from build123d import *

# Parameters (mm, degrees)
SKETCH2_R           = 6
SKETCH4_R           = 8
BOSS_EXTRUDE1_DEPTH = 2
SKETCH5_R           = 8
SKETCH5_R_2         = 6
BOSS_EXTRUDE2_DEPTH = 2


with BuildPart() as part:
    # Sweep1: sweep along a curve in space
    with BuildLine() as sweep1_path:
        Line((0, 0, 0), (0, 0, 20))
        ThreePointArc((-10, 0, 30), (-2.928932188, 0, 27.071067812), (0, 0, 20))
        Line((-10, 0, 30), (-96, 0, 30))
    # Sketch2 → Sweep1 (sweep)
    with BuildSketch(Plane.XY):
        Circle(SKETCH2_R)
    sweep(path=sweep1_path.line)

    # Sketch4 → Boss-Extrude1 (add)
    with BuildSketch(Plane(origin=(0, 0, 0), x_dir=(-1, 0, 0), z_dir=(0, 0, -1))):
        Circle(SKETCH4_R)
    extrude(amount=BOSS_EXTRUDE1_DEPTH)

    # Sketch5 → Boss-Extrude2 (add)
    with BuildSketch(Plane(origin=(0, 0, 6), x_dir=(-1, 0, 0), z_dir=(0, 0, -1))):
        Circle(SKETCH5_R)
        with Locations(Location((0, 0, 0), (0, 0, 180))):
            Circle(SKETCH5_R_2, mode=Mode.SUBTRACT)
    extrude(amount=BOSS_EXTRUDE2_DEPTH)


solid = part.part
Geometry check sheet. Reference: the model listing, model coordinates, mm. A direction names the side the tool comes from. Round coordinates to 2 decimals unless told otherwise and drop trailing zeros. Order: outer loops, then holes, each group sorted by start corner. A loop starts at its lowest first (then second) coordinate and runs counter-clockwise, first axis right, second up. Notation, with made-up numbers: (7.25, 62.25) - (51.25, 62.25) arc R13 ccw to (51.25, 66.25) - close; hole circle Ø7 at (-22, -39). An arc over 180 degrees is marked (long way). One line per question, with ' | ' between items. Start each with the question number.
(1) Sectioned sample at B-B on x = -37. Record the cut outline in (y, z).
(2) Thickness scan on L1, parallel to Z at x = -20, y = -0.5; L2, parallel to Z at x = -43, y = -4; L3, parallel to Y at x = -7, z = 5. Record the ranges inside material, lowest first. Write a range as [from, to].
(3) Depth check by flat-ended pin: pin 1 Ø1 at (x, y) = (-10.5, 2.5) entering from +Z; pin 2 Ø1 at (x, z) = (-61.5, 25.5) entering from +Y; pin 3 Ø8 at (x, y) = (3, 3.5) entering from +Z. Enter the tip coordinate at first touch or a pass-through.
(4) Sectioned sample at A-A on y = 0. Record the cut outline in (x, z), and give its area (3 significant figures).
(5) Release check for a two-part mould opening along Z. For faces 5 (the cylindrical face through (1.73, -7.81, -0.99)), 6 (the flat face through (0, 0, -2)), 7 (the cylindrical face through (-6, 0, 2)) record: released by +Z, released by -Z, zero draft, split by the parting line, or undercut.
(6) Sectioned sample at C-C on z = 7. Record the cut outline in (x, y), and give its area (3 significant figures).
(7) Access from +Z, -Z, +X, -X, +Y, -Y to the whole of each face (thin tool, end or side, straight path). Record for faces 1 (the flat face through (-96, 0, 30)), 2 (the cylindrical face through (1.73, -7.81, 5.01)), 3 (the cylindrical face through (-6, 0, 13)), 4 (the cylindrical face through (-54, 0, 24)).
Conclusion:
1) outline: circle Ø12 at (0, 30)
2) L1: z = [24.02, 35.98] | L2: z = [25.53, 34.47] | L3: y = [-3.87, 3.87]
3) pin 1: stops at z = 35.66 | pin 2: stops at y = 4.47 | pin 3: stops at z = 32.62
4) outline: (-96, 24) - (-10, 24) arc R4 cw to (-6, 20) - (-6, 6) - (-8, 6) - (-8, 4) - (-6, 4) - (-6, 0) - (-8, 0) - (-8, -2) - (8, -2) - (8, 0) - (6, 0) - (6, 4) - (8, 4) - (8, 6) - (6, 6) - (6, 20) arc R16 ccw to (-10, 36) - (-96, 36) - close | area: 1,500 mm2
5) face 5: zero draft | face 6: released by -Z | face 7: undercut
6) outline: circle Ø12 at (0, 0) | area: 113 mm2
7) face 1: +Z, -Z, -X, +Y, -Y | face 2: -Z | face 3: none | face 4: -X
